```python
from build123d import *

# Parameters (mm, degrees)
BOSS_EXTRUDE1_DEPTH     = 4.7498
CUT_EXTRUDE4_DEPTH      = 57.268848798
CUT_EXTRUDE4_DEPTH_BACK = 57.268848798
SKETCH1_4_R             = 4.064
SKETCH1_4_R_2           = 1.016


with BuildPart() as part:
    # Sketch1 → Boss-Extrude1 (new body)
    with BuildSketch(Plane.XY):
        with BuildLine():
            Line((-45.517091875, 9.830015002), (-22.51075, 10.989907038))
            ThreePointArc((-22.51075, 10.989907038), (0, 11.557), (22.51075, 10.989907038))
            Line((22.51075, 10.989907038), (45.517091875, 9.830015002))
            ThreePointArc((45.517091875, 9.830015002), (54.864, 0), (45.517091875, -9.830015002))
            Line((45.517091875, -9.830015002), (22.51075, -10.989907038))
            ThreePointArc((22.51075, -10.989907038), (0, -11.557), (-22.51075, -10.989907038))
            Line((-22.51075, -10.989907038), (-45.517091875, -9.830015002))
            ThreePointArc((-45.517091875, -9.830015002), (-54.864, 0), (-45.517091875, 9.830015002))
        make_face()
    extrude(amount=BOSS_EXTRUDE1_DEPTH)

    # Sketch1<4> → Cut-Extrude4 (cut, two sides: drawn at the far end of the back side and taken through both)
    with BuildSketch(Plane.XY.offset(-CUT_EXTRUDE4_DEPTH_BACK)):
        with Locations((-45.0215, 0)):
            Circle(SKETCH1_4_R)
        with Locations((-45.0215, 6.985)):
            Circle(SKETCH1_4_R_2)
        with Locations((-52.0065, 0)):
            Circle(SKETCH1_4_R_2)
        with Locations((-38.0365, 0)):
            Circle(SKETCH1_4_R_2)
        with Locations((-45.0215, -6.985)):
            Circle(SKETCH1_4_R_2)
        with Locations((45.0215, 0)):
            Circle(SKETCH1_4_R)
        with Locations((45.0215, 6.985)):
            Circle(SKETCH1_4_R_2)
        with Locations((52.0065, 0)):
            Circle(SKETCH1_4_R_2)
        with Locations((45.0215, -6.985)):
            Circle(SKETCH1_4_R_2)
        with Locations((38.0365, 0)):
            Circle(SKETCH1_4_R_2)
    extrude(amount=CUT_EXTRUDE4_DEPTH + CUT_EXTRUDE4_DEPTH_BACK, mode=Mode.SUBTRACT)


solid = part.part
```
Verification items for the finished model (mm, model axes). Coordinates: 2 decimals unless noted, no trailing zeros. Loops run counter-clockwise (first coordinate to the right, second up) from the corner with the lowest first, then second, coordinate; pieces in that order, holes last. Notation, with made-up numbers: (81.25, -11.5) - (117.25, -11.5) arc R13 ccw to (117.25, 2.5) - close; hole circle Ø3 at (22, -9.75). An arc over 180 degrees is marked (long way). Answer as a JSON object with one key per item and string values.
(1) Go/stop test with flat-tipped pins: pin 1 Ø1.8 at (x, y) = (45.02, -6.98) entering from +Z; pin 2 Ø2 at (y, z) = (7.5, 0.5) entering from -X; pin 3 Ø2 at (y, z) = (7.5, 3) entering from +X. Record where each tip stops, or that it passes through.
Response:
{"pin 1": "passes through", "pin 2": "stops at x = -52.41", "pin 3": "stops at x = 52.41"}
(2) Cross-section at C-C, the plane z = 4. Count the separate pieces of the cut face and the enclosed holes in it, then the cut area to 3 significant figures.
Response:
{"separate pieces": "1", "enclosed holes": "10", "area": "2,140 mm²"}
(3) Cross-section at A-A, the plane y = 0. Record the boundary of the cut face in (x, z), then the cut area to 3 significant figures.
Response:
{"outline": "(-54.86, 0) - (-53.02, 0) - (-53.02, 4.75) - (-54.86, 4.75) - close; (-50.99, 0) - (-49.09, 0) - (-49.09, 4.75) - (-50.99, 4.75) - close; (-40.96, 0) - (-39.05, 0) - (-39.05, 4.75) - (-40.96, 4.75) - close; (-37.02, 0) - (37.02, 0) - (37.02, 4.75) - (-37.02, 4.75) - close; (39.05, 0) - (40.96, 0) - (40.96, 4.75) - (39.05, 4.75) - close; (49.09, 0) - (50.99, 0) - (50.99, 4.75) - (49.09, 4.75) - close; (53.02, 0) - (54.86, 0) - (54.86, 4.75) - (53.02, 4.75) - close", "area": "405 mm²"}
(4) Scan lines: line 1 along X through (y, z) = (3, 2.6); line 2 along X through (y, z) = (7.75, 4.1); line 3 along Y through (x, z) = (3, 0.5). Record each from-to range of solid material in increasing order.
Response:
{"line 1": "x = -54.4 to -47.76, -42.28 to 42.28, 47.76 to 54.4", "line 2": "x = -51.09 to -45.69, -44.35 to 44.35, 45.69 to 51.09", "line 3": "y = -11.55 to 11.55"}
(5) Mould release check, pull along X, two halves, no side actions. Record for faces 1 (the cylindrical face through (-54.86, -0.21, 2.34)), 2 (the cylindrical face through (50.99, 0.04, 2.34)), 3 (the flat face through (34.2, -10.4, 2.3)), 4 (the flat face through (1, 0, 4.75)): pulls with the +X half, pulls with the -X half, needs draft (parallel to the pull), parting line crosses it, or undercut.
Response:
{"face 1": "pulls with the -X half", "face 2": "undercut", "face 3": "pulls with the +X half", "face 4": "needs draft"}
(6) Cross-section at D-D, the plane x = -19. Record the boundary of the cut face in (y, z), then the cut area to 3 significant figures.
Response:
{"outline": "(-11.15, 0) - (11.15, 0) - (11.15, 4.75) - (-11.15, 4.75) - close", "area": "106 mm²"}
(7) Cross-section at B-B, the plane x = -47. Record the boundary of the cut face in (y, z).
Response:
{"outline": "(-9.64, 0) - (-3.55, 0) - (-3.55, 4.75) - (-9.64, 4.75) - close; (3.55, 0) - (9.64, 0) - (9.64, 4.75) - (3.55, 4.75) - close"}
